Check sheet for the modelled part. Datum: model origin and axes. Units: mm. A direction names the side the tool comes from. Give positions to 0.01 mm unless a question says otherwise; leave off trailing zeros. Write each loop counter-clockwise with the first axis right and the second up, starting at its lowest first coordinate (ties: lowest second). Pieces come first, ordered by that corner, then holes. Notation, with made-up numbers: (82.5, 52.25) -> (127.5, 52.25) arc R25 cw to (127.5, 89.25) -> close; hole circle Ø2 at (78.5, -34.75). An arc over 180 degrees is marked (long way). Use a Markdown table: item, result. Add a question column.
1. Release check for a two-part mould opening along Y. For faces 1 (the flat face through (65, 5, 20)), 2 (the conical face through (0.313, 9.149, 4.759)), 3 (the flat face through (0, 0, 0)) record: released by +Y, released by -Y, zero draft, split by the parting line, or undercut.
2. Scan lines: probe 1 along X at (y, z) = (-17.5, 14); probe 2 along Y at (x, z) = (32.5, 0); probe 3 along Z at (x, y) = (26.5, 1). Record each from-to range of solid material in increasing order. Write a range as [from, to].
3. Cross-section at D-D (x = 47). Enter the section's corners in (y, z).
4. Cross-section at A-A (z = 0). Enter the section's corners in (x, y).
5. Cross-section at B-B (y = 0). Enter the section's corners in (x, z).
6. Gauge pin test, flat ends, axial feed: P1, Ø2, axis at x = 44, z = -12, coming from the +Y side; P2, Ø10, axis at x = 29, z = 6, coming from the -Y side; P3, Ø12, axis at x = 66.5, y = -16, coming from the -Z side. Record the tip position at first contact, or that the pin passes through.
7. Set-up check for faces 4 (the cylindrical face through (114.72, -0.66, -14.985)), 5 (the flat face through (65, 0, 18.5)), 6 (the flat face through (175, 0, 0)), 7 (the cylindrical face through (64.58, -0.92, -22.48)), 8 (the flat face through (35, -0.3, -15.4)): record each of +Z, -Z, +X, -X, +Y, -Y from which the full face is reachable in a straight line by a thin tool's end or side.
8. Cross-section at C-C (x = 19.5). Enter the section's corners in (y, z), then the cut area to 3 significant figures.
from build123d import *

# Parameters (mm, degrees)
F4_DEPTH = 60


with BuildPart() as f2:
    # F0 (on Front) → F2 (revolve)
    with BuildSketch(Plane.XZ):
        Polygon((0, 15), (0, 0), (175, 0), (175, 10), (135, 15), (95, 15), (95, 22.5), (35, 22.5), (35, 15), align=None)
    revolve(axis=Axis((109.590694, 0, 0), (1, 0, 0)))

    # F3 (on face) → F4 (cut, through all)
    with BuildSketch(Plane.YZ.offset(95)):
        with BuildLine():
            ThreePointArc((5, 21.937411), (2.515776, 22.35891), (0, 22.5))
            ThreePointArc((0, 22.5), (-2.515776, 22.35891), (-5, 21.937411))
            Line((-5, 21.937411), (-5, 18.5))
            Line((-5, 18.5), (5, 18.5))
            Line((5, 18.5), (5, 21.937411))
        make_face()
    extrude(amount=-F4_DEPTH, mode=Mode.SUBTRACT)

    # F5 (on Front) → F6 (revolve, cut)
    with BuildSketch(Plane.XZ):
        Polygon((5, 15), (0, 15), (0, 10), align=None)
    revolve(axis=Axis((109.590694, 0, 0), (1, 0, 0)), mode=Mode.SUBTRACT)


solid = f2.part
Worked answers:
| question | item | result |
|---|---|---|
| 1 | face 1 | undercut |
| 1 | face 2 | split by the parting line |
| 1 | face 3 | zero draft |
| 2 | probe 1 | x = [35, 95] |
| 2 | probe 2 | y = [-15, 15] |
| 2 | probe 3 | z = [-14.97, 14.97] |
| 3 | outline | (-5, 18.5) -> (-5, 21.94) arc R22.5 ccw (long way) to (5, 21.94) -> (5, 18.5) -> close |
| 4 | outline | (0, -10) -> (5, -15) -> (35, -15) -> (35, -22.5) -> (95, -22.5) -> (95, -15) -> (135, -15) -> (175, -10) -> (175, 10) -> (135, 15) -> (95, 15) -> (95, 22.5) -> (35, 22.5) -> (35, 15) -> (5, 15) -> (0, 10) -> close |
| 5 | outline | (0, -10) -> (5, -15) -> (35, -15) -> (35, -22.5) -> (95, -22.5) -> (95, -15) -> (135, -15) -> (175, -10) -> (175, 10) -> (135, 15) -> (95, 15) -> (95, 18.5) -> (35, 18.5) -> (35, 15) -> (5, 15) -> (0, 10) -> close |
| 6 | P1 | stops at y = 19.63 |
| 6 | P2 | stops at y = -14.97 |
| 6 | P3 | stops at z = -20.16 |
| 7 | face 4 | +X |
| 7 | face 5 | +Z, +X, -X |
| 7 | face 6 | +Z, -Z, +X, +Y, -Y |
| 7 | face 7 | +X, -X |
| 7 | face 8 | -X |
| 8 | outline | circle Ø30 at (0, 0) |
| 8 | area | 707 mm² |
